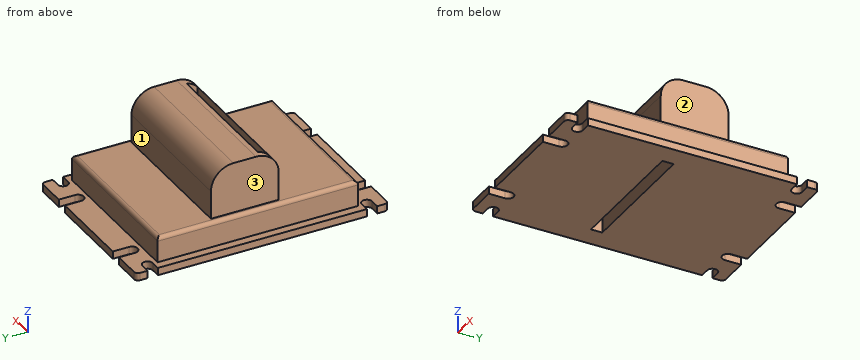
```python
from build123d import *

# Parameters (mm, degrees)
SKETCH1_W           = 93
SKETCH1_H           = 134
BOSS_EXTRUDE1_DEPTH = 4
SKETCH2_W           = 88
SKETCH2_H           = 106.5
BOSS_EXTRUDE2_DEPTH = 13.5
FILLET2_R           = 2
SKETCH5_W           = 78
SKETCH5_H           = 36
BOSS_EXTRUDE3_DEPTH = 27
FILLET3_R           = 12
SKETCH6_W           = 70
SKETCH6_H           = 6
CUT_EXTRUDE1_DEPTH  = 45.5
SKETCH9_R           = 2.75
SKETCH9_W           = 5
SKETCH9_H           = 5.5
CUT_EXTRUDE3_DEPTH  = 10
CUT_EXTRUDE6_DEPTH  = 10
SKETCH13_W          = 2
SKETCH13_H          = 106.5
CUT_EXTRUDE7_DEPTH  = 13.5
FILLET4_R           = 2


with BuildPart() as part:
    # Sketch1 → Boss-Extrude1 (new body)
    with BuildSketch(Plane.XY):
        Rectangle(SKETCH1_W, SKETCH1_H)
    extrude(amount=BOSS_EXTRUDE1_DEPTH)

    # Sketch2 → Boss-Extrude2 (add)
    with BuildSketch(Plane.XY.offset(4)):
        Rectangle(SKETCH2_W, SKETCH2_H)
    extrude(amount=BOSS_EXTRUDE2_DEPTH)

    # Fillet2
    fillet2_edges = [part.edges().sort_by_distance(p)[0] for p in [
        (46.5, -67, 2),
        (-46.5, -67, 2),
        (-46.5, 67, 2),
        (46.5, 67, 2),
    ]]
    fillet(fillet2_edges, radius=FILLET2_R)

    # Sketch5 → Boss-Extrude3 (add)
    with BuildSketch(Plane.XY.offset(17.5)):
        with Locations((0, 5.25)):
            Rectangle(SKETCH5_W, SKETCH5_H)
    extrude(amount=BOSS_EXTRUDE3_DEPTH)

    # Fillet3
    fillet3_edges = [part.edges().sort_by_distance(p)[0] for p in [
        (0, 23.25, 44.5),
        (0, -12.75, 44.5),
    ]]
    fillet(fillet3_edges, radius=FILLET3_R)

    # Sketch6 → Cut-Extrude1 (cut, through all)
    with BuildSketch(Plane.XY.offset(44.5)):
        with Locations((0, -6.75)):
            Rectangle(SKETCH6_W, SKETCH6_H)
    extrude(amount=-CUT_EXTRUDE1_DEPTH, mode=Mode.SUBTRACT)

    # Sketch9 → Cut-Extrude3 (cut)
    with BuildSketch(Plane.XY.offset(4)):
        with Locations((41.5, 58.25)):
            Circle(SKETCH9_R)
        with Locations((-41.5, 58.25)):
            Circle(SKETCH9_R)
        with Locations((-41.5, -58.25)):
            Circle(SKETCH9_R)
        with Locations((41.5, -58.25)):
            Circle(SKETCH9_R)
        with Locations((44, 58.25)):
            Rectangle(SKETCH9_W, SKETCH9_H)
        with Locations((-44, 58.25)):
            Rectangle(SKETCH9_W, SKETCH9_H)
        with Locations((-44, -58.25)):
            Rectangle(SKETCH9_W, SKETCH9_H)
        with Locations((44, -58.25)):
            Rectangle(SKETCH9_W, SKETCH9_H)
    extrude(amount=-CUT_EXTRUDE3_DEPTH, mode=Mode.SUBTRACT)

    # Sketch8 → Cut-Extrude6 (cut)
    with BuildSketch(Plane.XY.offset(4)):
        with BuildLine():
            Line((29.5, 67), (23.5, 67))
            Line((23.5, 67), (23.5, 58.4))
            ThreePointArc((23.5, 58.4), (26.5, 55.4), (29.5, 58.4))
            Line((29.5, 58.4), (29.5, 67))
        make_face()
        with BuildLine():
            ThreePointArc((-29.5, 58.4), (-26.5, 55.4), (-23.5, 58.4))
            Line((-23.5, 58.4), (-23.5, 67))
            Line((-23.5, 67), (-29.5, 67))
            Line((-29.5, 67), (-29.5, 58.4))
        make_face()
        with BuildLine():
            Line((-29.5, -67), (-23.5, -67))
            Line((-23.5, -67), (-23.5, -58.4))
            ThreePointArc((-23.5, -58.4), (-26.5, -55.4), (-29.5, -58.4))
            Line((-29.5, -58.4), (-29.5, -67))
        make_face()
        with BuildLine():
            ThreePointArc((29.5, -58.4), (26.5, -55.4), (23.5, -58.4))
            Line((23.5, -58.4), (23.5, -67))
            Line((23.5, -67), (29.5, -67))
            Line((29.5, -67), (29.5, -58.4))
        make_face()
    extrude(amount=-CUT_EXTRUDE6_DEPTH, mode=Mode.SUBTRACT)

    # Sketch13 → Cut-Extrude7 (cut)
    with BuildSketch(Plane.XY.offset(17.5)):
        with Locations((-43, 0)):
            Rectangle(SKETCH13_W, SKETCH13_H)
        with Locations((43, 0)):
            Rectangle(SKETCH13_W, SKETCH13_H)
    extrude(amount=-CUT_EXTRUDE7_DEPTH, mode=Mode.SUBTRACT)

    # Fillet4
    fillet4_edges = [part.edges().sort_by_distance(p)[0] for p in [
        (0, 53.25, 17.5),
        (0, -53.25, 17.5),
        (-42, 0, 17.5),
        (42, 0, 17.5),
    ]]
    fillet(fillet4_edges, radius=FILLET4_R)


solid = part.part
```
The listing builds one solid part. Answer for the finished solid, in the listing's coordinates (mm). Face numbers are marked on the shaded views. A direction names the side the tool comes from. Give positions to 0.01 mm unless a question says otherwise; leave off trailing zeros. Loops run counter-clockwise (first coordinate to the right, second up) from the corner with the lowest first, then second, coordinate; pieces in that order, holes last. Notation, with made-up numbers: M 68,33.5 L 102,33.5 A13 cw 102,46.5 Z; hole C 52.25,33.25 d2. An arc over 180 degrees is marked long. One line per item, written item: value.
Q1. Flat-ended cylindrical pins translate along their axes: P1, Ø1, axis at x = -18.5, z = 30.5, coming from the -Y side; P2, Ø8, axis at y = -1.5, z = 35.5, coming from the +X side; P3, Ø6.5, axis at y = -6.5, z = 16.5, coming from the -X side. Find the tip coordinate at first contact, or state that the pin passes through.
Working result:
P1: stops at y = -12.75
P2: stops at x = 39
P3: stops at x = -42
Q2. A cutting plane is placed at B-B on z = 10.5. Determine the outline of the cut face in (x, y).
Working result:
outline: M -42,-53.25 L 42,-53.25 L 42,53.25 L -42,53.25 Z; hole M -35,-9.75 L 35,-9.75 L 35,-3.75 L -35,-3.75 Z
Q3. For the marked faces 1, 2 and 3, determine the directions among +Z, -Z, +X, -X, +Y, -Y from which every point of the face is accessible in a straight line to the end or side of a thin tool.
Working result:
face 1: +Z, +X, -X, +Y
face 2: +Z, +X, +Y, -Y
face 3: +Z, -X, +Y, -Y
Q4. A cutting plane is placed at A-A on x = -5. Determine the outline of the cut face in (y, z).
Working result:
outline: M -67,0 L -9.75,0 L -9.75,40.44 A12 ccw -12.75,32.5 L -12.75,17.5 L -51.25,17.5 A2 ccw -53.25,15.5 L -53.25,4 L -67,4 Z; M -3.75,0 L 67,0 L 67,4 L 53.25,4 L 53.25,15.5 A2 ccw 51.25,17.5 L 23.25,17.5 L 23.25,32.5 A12 ccw 11.25,44.5 L -0.75,44.5 A12 ccw -3.75,44.12 Z
Q5. A cutting plane is placed at C-C on x = 26.5. Determine the outline of the cut face in (y, z), then the cut area to 3 significant figures.
Working result:
outline: M -55.4,0 L -9.75,0 L -9.75,40.44 A12 ccw -12.75,32.5 L -12.75,17.5 L -51.25,17.5 A2 ccw -53.25,15.5 L -53.25,4 L -55.4,4 Z; M -3.75,0 L 55.4,0 L 55.4,4 L 53.25,4 L 53.25,15.5 A2 ccw 51.25,17.5 L 23.25,17.5 L 23.25,32.5 A12 ccw 11.25,44.5 L -0.75,44.5 A12 ccw -3.75,44.12 Z
area: 2,530 mm^2
Q6. Find the intervals of material crossed by line 1 (Y direction, x = -2.5, z = 12); line 2 (Y direction, x = 18.5, z = 3); line 3 (Z direction, x = 30, y = -59), in increasing order. Write a range as from..to.
Working result:
line 1: y = -53.25..-9.75, -3.75..53.25
line 2: y = -67..-9.75, -3.75..67
line 3: z = 0..4
